```python
from build123d import *

# Parameters (mm, degrees)
EXTRUDE_1_DEPTH = 2.2
FILLET_1_R      = 4


with BuildPart() as part:
    # 草图1 → 凸台-拉伸1 (new body)
    with BuildSketch(Plane.XY):
        Polygon((10.6, 4.15), (-9.6, 4.15), (-21.05, -5.5), (-21.05, -20.7), (-11.05, -20.7), (10.6, -2.45349345), align=None)
        with BuildLine():
            ThreePointArc((-14.245, -16.695), (-14.539357685, -17.405642315), (-15.25, -17.7))
            Line((-15.25, -17.7), (-17.55, -17.7))
            ThreePointArc((-17.55, -17.7), (-18.555, -16.695), (-17.55, -15.69))
            Line((-17.55, -15.69), (-17.55, -9.51))
            ThreePointArc((-17.55, -9.51), (-18.555, -8.505), (-17.55, -7.5))
            Line((-17.55, -7.5), (-15.25, -7.5))
            ThreePointArc((-15.25, -7.5), (-14.539357685, -7.794357685), (-14.245, -8.505))
            ThreePointArc((-14.245, -8.505), (-14.539357685, -9.215642315), (-15.25, -9.51))
            Line((-15.25, -9.51), (-15.25, -15.69))
            ThreePointArc((-15.25, -15.69), (-14.539357685, -15.984357685), (-14.245, -16.695))
        make_face(mode=Mode.SUBTRACT)
        with BuildLine():
            Line((5.59, -1.15), (-5.59, -1.15))
            ThreePointArc((-5.59, -1.15), (-6.595, -2.155), (-7.6, -1.15))
            Line((-7.6, -1.15), (-7.6, 1.15))
            ThreePointArc((-7.6, 1.15), (-6.595, 2.155), (-5.59, 1.15))
            Line((-5.59, 1.15), (5.59, 1.15))
            ThreePointArc((5.59, 1.15), (6.595, 2.155), (7.6, 1.15))
            Line((7.6, 1.15), (7.6, -1.15))
            ThreePointArc((7.6, -1.15), (6.595, -2.155), (5.59, -1.15))
        make_face(mode=Mode.SUBTRACT)
    extrude(amount=EXTRUDE_1_DEPTH)

    # 圆角1
    fillet_1_edges = [part.edges().sort_by_distance(p)[0] for p in [
        (-9.6, 4.15, 1.1),
        (10.6, 4.15, 1.1),
        (10.6, -2.45349345, 1.1),
        (-11.05, -20.7, 1.1),
        (-21.05, -20.7, 1.1),
        (-21.05, -5.5, 1.1),
    ]]
    fillet(fillet_1_edges, radius=FILLET_1_R)


solid = part.part
```
Geometry check sheet. Reference: the model listing, model coordinates, mm. A direction names the side the tool comes from. Round coordinates to 2 decimals unless told otherwise and drop trailing zeros. Loops run counter-clockwise (first coordinate to the right, second up) from the corner with the lowest first, then second, coordinate; pieces in that order, holes last. Notation, with made-up numbers: (87.25, -28.5) - (143.25, -28.5) arc R27 cw to (143.25, 1.5) - close; hole circle Ø4 at (32.25, 52.5). An arc over 180 degrees is marked (long way). Use a Markdown table: item, result.
Q1. Cross-section at C-C on x = -16. Record the cut outline in (y, z).
Solutions:
| item | result |
|---|---|
| outline | (-20.7, 0) - (-17.7, 0) - (-17.7, 2.2) - (-20.7, 2.2) - close; (-7.5, 0) - (-1.24, 0) - (-1.24, 2.2) - (-7.5, 2.2) - close |
Q2. Material ranges on line 1 (X direction, y = 1.25, z = 1.8); line 2 (Y direction, x = -6, z = 0.25); line 3 (X direction, y = -15.5, z = 1.4), recorded low to high.
Solutions:
| item | result |
|---|---|
| line 1 | x = -13.04 to -7.6, -5.59 to 5.59, 7.6 to 10.45 |
| line 2 | y = -16.44 to -1.96, 1.96 to 4.15 |
| line 3 | x = -21.05 to -17.55, -15.25 to -4.88 |
Q3. Cross-section at A-A on z = 1.35. Record the cut outline in (x, y) (3 decimals), plus the area to 3 significant figures.
Solutions:
| item | result |
|---|---|
| outline | (-21.05, -16.7) arc R4 ccw to (-17.05, -20.7) - (-12.511, -20.7) arc R4 ccw to (-9.933, -19.759) - (9.178, -3.652) arc R4 ccw to (10.6, -0.594) - (10.6, 0.15) arc R4 ccw to (6.6, 4.15) - (-8.139, 4.15) arc R4 ccw to (-10.717, 3.209) - (-19.628, -4.301) arc R4 ccw to (-21.05, -7.36) - close; hole (-17.55, -17.7) - (-15.25, -17.7) arc R1.005 ccw to (-15.25, -15.69) - (-15.25, -9.51) arc R1.005 ccw to (-15.25, -7.5) - (-17.55, -7.5) arc R1.005 ccw to (-17.55, -9.51) - (-17.55, -15.69) arc R1.005 ccw to start; hole (-7.6, -1.15) arc R1.005 ccw to (-5.59, -1.15) - (5.59, -1.15) arc R1.005 ccw to (7.6, -1.15) - (7.6, 1.15) arc R1.005 ccw to (5.59, 1.15) - (-5.59, 1.15) arc R1.005 ccw to (-7.6, 1.15) - close |
| area | 454 mm2 |
Q4. Access from +Z, -Z, +X, -X, +Y, -Y to the whole of each face (thin tool, end or side, straight path). Record for faces 4 (the cylindrical face through (-19.909, -19.497, 1.115)), 5 (the flat face through (-16, -17.7, 1)).
Solutions:
| item | result |
|---|---|
| face 4 | +Z, -Z, -X, -Y |
| face 5 | +Z, -Z |
Q5. Go/stop test with flat-tipped pins: P1, Ø4, axis at x = -17.5, y = -14.5, coming from the +Z side; P2, Ø1.1, axis at y = 0, z = 1.5, coming from the -X side; P3, Ø0.7, axis at y = -14, z = 0.5, coming from the +X side (3 decimals). Record where each tip stops, or that it passes through.
Solutions:
| item | result |
|---|---|
| P1 | stops at z = 2.2 |
| P2 | stops at x = -15.18 |
| P3 | stops at x = -2.685 |
Q6. Cross-section at D-D on x = -12. Record the cut outline in (y, z), plus the area to 3 significant figures.
Solutions:
| item | result |
|---|---|
| outline | (-20.67, 0) - (2.13, 0) - (2.13, 2.2) - (-20.67, 2.2) - close |
| area | 50.1 mm2 |
Q7. Cross-section at B-B on x = -1. Record the cut outline in (y, z), plus the area to 3 significant figures.
Solutions:
| item | result |
|---|---|
| outline | (-12.23, 0) - (-1.15, 0) - (-1.15, 2.2) - (-12.23, 2.2) - close; (1.15, 0) - (4.15, 0) - (4.15, 2.2) - (1.15, 2.2) - close |
| area | 31.0 mm2 |
Q8. Draft check along Y on faces 1 (the cylindrical face through (9.397, 3.009, 1.115)), 2 (the cylindrical face through (-6.617, 2.155, 1.085)), 3 (the cylindrical face through (-11.12, -20.45, 1.12)). Enter one of: released by +Y, released by -Y, zero draft, split by the parting line, or undercut.
Solutions:
| item | result |
|---|---|
| face 1 | released by +Y |
| face 2 | undercut |
| face 3 | released by -Y |
